```python
from build123d import *

# Parameters (mm, degrees)
CROQUIS1_R              = 1.25
SALIENTE_EXTRUIR1_DEPTH = 2.4


with BuildPart() as part:
    # Croquis1 → Saliente-Extruir1 (new body)
    with BuildSketch(Plane(origin=(0, 0, 0), x_dir=(1, 0, 0), z_dir=(0, 1, 0))):
        Polygon((-1.58771324, 2.75), (-3.175426481, 0), (-1.58771324, -2.75), (1.58771324, -2.75), (3.175426481, 0), (1.58771324, 2.75), align=None)
        Circle(CROQUIS1_R, mode=Mode.SUBTRACT)
    extrude(amount=SALIENTE_EXTRUIR1_DEPTH)

    # Croquis3 one side → Revolución2 (revolve)
    with BuildSketch(Plane(origin=(0, 0, 0), x_dir=(0, 0, -1), z_dir=(1, 0, 0))):
        with BuildLine():
            Line((0, 6), (0, 2.4))
            Line((0, 2.4), (2.75, 2.4))
            ThreePointArc((2.75, 2.4), (2.265088298, 4.879928561), (0, 6))
        make_face()
    revolve(axis=Axis((0, 6, 0), (0, -1, 0)))


solid = part.part
```
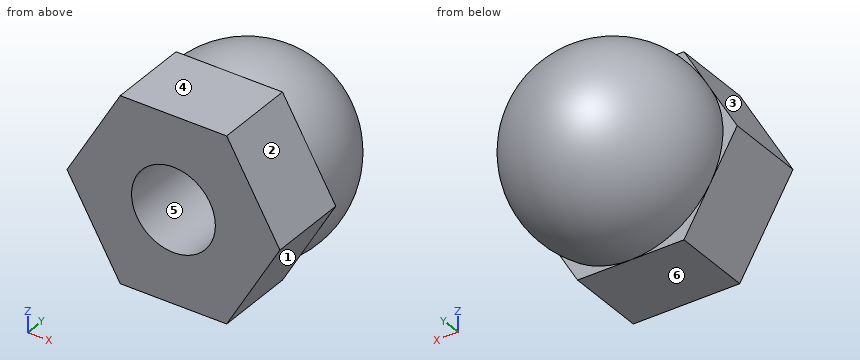
Input: part model. Units: mm. Frame: model coordinates. Face numbers are marked on the shaded views. A direction names the side the tool comes from. Coordinates: 2 decimals unless noted, no trailing zeros. Loops run counter-clockwise (first coordinate to the right, second up) from the corner with the lowest first, then second, coordinate; pieces in that order, holes last.
Q1. Section B-B, the plane z = -0.4. Return the cut outline in (x, y), and give its area (3 significant figures).
Results are:
outline: (-2.94, 0) - (-1.18, 0) - (-1.18, 2.4) - (1.18, 2.4) - (1.18, 0) - (2.94, 0) - (2.94, 2.4) - (2.72, 2.4) arc R2.82 ccw (long way) to (-2.72, 2.4) - (-2.94, 2.4) - close
area: 25.1 mm2
Q2. Section C-C, the plane y = 4.65. Return the cut outline in (x, z), and give its area (3 significant figures).
Results are:
outline: circle Ø4.85 at (0, 0)
area: 18.5 mm2
Q3. Mould query, pull axis Z, two halves, no side actions, for the marked faces 4, 5 and 6. Classes: +Z half, -Z half, draft (parallel to the pull), parting line (faces both ways), or undercut.
Results are:
face 4: +Z half
face 5: undercut
face 6: -Z half
Q4. Set-up query: the marked faces 1, 2 and 3. Return all of +Z, -Z, +X, -X, +Y, -Y with unobstructed straight access to the full face (end or side cutting, diameter ignored); none if empty.
Results are:
face 1: -Z, +X, -Y
face 2: +Z, +X, -Y
face 3: +Z, -X, -Y
Q5. Contact query for flat-ended pins moving along their axis: pin 1 (1.2 mm diameter, centred on x = 0, y = 1.5, fed in from -Z); pin 2 (1.1 mm diameter, centred on x = 1.5, z = 2.5, fed in from +Y); pin 3 (1 mm diameter, centred on x = 1.5, y = 1.5, fed in from +Z); pin 4 (3 mm diameter, centred on x = -0.5, z = 0, fed in from -Y). Output: stop coordinate, or through.
Results are:
pin 1: stops at z = -2.75
pin 2: stops at y = 4.74
pin 3: stops at z = 2.75
pin 4: stops at y = 0
Q6. Line query: line 1 along Z through (x, y) = (0, 1.35); line 2 along X through (y, z) = (0.9, -0.05); line 3 along X through (y, z) = (1.8, -0.75). Output: solid intervals per line, ascending.
Results are:
line 1: z = -2.75 to -1.25, 1.25 to 2.75
line 2: x = -3.15 to -1.25, 1.25 to 3.15
line 3: x = -2.74 to -1, 1 to 2.74
Q7. Section A-A, the plane x = 0.75. Return the cut outline in (y, z), and give its area (3 significant figures).
Results are:
outline: (0, -2.75) - (2.4, -2.75) - (2.4, -2.65) arc R2.75 ccw (long way) to (2.4, 2.65) - (2.4, 2.75) - (0, 2.75) - (0, 1) - (2.4, 1) - (2.4, -1) - (0, -1) - close
area: 24.3 mm2
